Input: part model. Units: mm. Frame: model coordinates. Face numbers are marked on the shaded views. A direction names the side the tool comes from. Give positions to 0.01 mm unless a question says otherwise; leave off trailing zeros. Loops run counter-clockwise (first coordinate to the right, second up) from the corner with the lowest first, then second, coordinate; pieces in that order, holes last. Notation, with made-up numbers: M 41,56.25 L 71,56.25 A13 ccw 71,69.25 Z; hole C 79,-7 d3. An arc over 180 degrees is marked long. Return JSON: item names as keys, results as strings. Group by question number.
Autodesk Inventor part; units mm, degrees
ref_plane "YZ Plane" through (0, 0, 0) normal (1, 0, 0) x (0, 1, 0)
ref_plane "XZ Plane" through (0, 0, 0) normal (0, 1, 0) x (-1, 0, 0)
ref_plane "XY Plane" through (0, 0, 0) normal (0, 0, 1) x (1, 0, 0)
sketch "Sketch1" plane through (0, 0, 0) normal (0, 1, 0) x (-1, 0, 0)
  circle A0 centre (19.9072, 0) radius 5
  line L0 (-15.0928, 12) -> (34.9072, 12)
  line L1 (34.9072, 12) -> (34.9072, -12)
  line L2 (34.9072, -12) -> (-15.0928, -12)
  line L3 (-15.0928, -12) -> (-15.0928, 12)
  point P0 (0, 0)
  dimension "d0" = 10
  dimension "d1" = 12
  dimension "d2" = 24
  dimension "d3" = 35
  dimension "d4" = 50
extrude "Extrusion1" add sketch "Sketch1" along normal blind 10
sketch "Sketch2" plane through (15.0928, 0, 12) normal (1, 0, 0) x (0, 0, -1)
  line L0 (12, 0) -> (12, -23) construction
  line L1 (12, -23) -> (-0.5, -23) construction
  circle A0 centre (-0.5, -23) radius 3
  line L2 (31, 10) -> (-7, 10)
  line L3 (-7, 10) -> (-7, -33)
  line L4 (-7, -33) -> (31, -33)
  line L5 (31, -33) -> (31, 10)
  line L6 (31, 10) -> (-7, -33) construction
  line L7 (-7, 10) -> (31, -33) construction
  circle A1 centre (24.5, -23) radius 3
  point P0 (12, -11.5)
  dimension "d7" = 6
  dimension "d8" = 12.5
extrude "Extrusion2" add sketch "Sketch2" against normal blind 10
chamfer "Chamfer1" distance 15 angle 45 1 edges at (5.0928, 0, 0)
sketch "Sketch3" plane through (-34.9072, 0, -12) normal (-1, 0, 0) x (0, 0, 1)
  circle A0 centre (12, 5) radius 2.95
  line L0 (0, 10) -> (24, 10)
  point P0 (12, 0)
  dimension "d14" = 5.9
  dimension "d15" = 5
extrude "Extrusion3" cut sketch "Sketch3" against normal blind 16
properties part number "Mitutoyo holder"
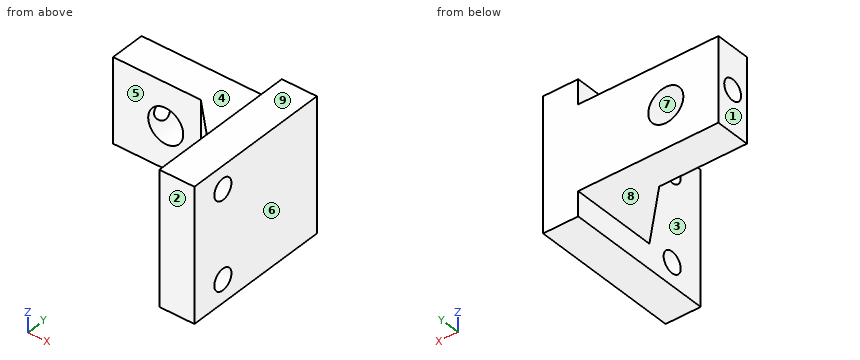
Item 1: Section A-A, the plane y = -23. Return loops of the section in (x, z).
Item 2: Section C-C, the plane z = 8. Return loops of the section in (x, y).
Item 3: Reachability of the marked faces 1, 2, 3, 4 and 5 from +Z, -Z, +X, -X, +Y, -Y: full face, straight path, thin tool, end or side. Return the list, or none.
Item 4: Material intervals for line 1 (Y direction, x = -27.25, z = 0); line 2 (Z direction, x = -31, y = 5); line 3 (Y direction, x = 10.5, z = -12.5), sorted ascending. Write a range as from..to.
Item 5: First-contact query: pin 1 Ø19 at (x, z) = (-18, 4) entering from -Y; pin 2 Ø20 at (x, y) = (-23.5, -6) entering from -Z; pin 3 Ø16 at (x, z) = (-19.91, 0) entering from -Y. Flat tips, straight axial feed; report the tip coordinate or a pass-through.
Item 6: Section B-B, the plane z = 14.5. Return loops of the section in (x, y), then the cut area to 3 significant figures.
Item 7: Section D-D, the plane z = -2. Return loops of the section in (x, y).
Item 8: Pull-direction query (Z, two-part tool) for the marked faces 6, 7, 8 and 9; classes: pulls with the +Z half, pulls with the -Z half, needs draft (parallel to the pull), parting line crosses it, or undercut.
Answer below:
{
 "1": {"outline": "M 5.09,-19 L 15.09,-19 L 15.09,-15.5 L 5.09,-15.5 Z; M 5.09,-9.5 L 15.09,-9.5 L 15.09,9.5 L 5.09,9.5 Z; M 5.09,15.5 L 15.09,15.5 L 15.09,19 L 5.09,19 Z"},
 "2": {"outline": "M -34.91,0 L -9.91,0 L 5.09,-15 L 5.09,-33 L 15.09,-33 L 15.09,10 L -34.91,10 Z"},
 "3": {"face 1": "+Z, -Z, -X, +Y, -Y", "face 2": "+Z, -Z, +X, -X, -Y", "face 3": "-X, -Y", "face 4": "+Z, -X, +Y, -Y", "face 5": "+Z, -Z, -X, -Y"},
 "4": {"line 1": "0..2.05, 7.95..10", "line 2": "-12..-2.95, 2.95..12", "line 3": "-33..-26, -20..10"},
 "5": {"pin 1": "y = -1.41", "pin 2": "z = -12", "pin 3": "y = 0"},
 "6": {"outline": "M 5.09,-33 L 15.09,-33 L 15.09,-25.24 L 5.09,-25.24 Z; M 5.09,-20.76 L 15.09,-20.76 L 15.09,10 L 5.09,10 Z", "area": "385 mm^2"},
 "7": {"outline": "M -34.91,0 L -24.49,0 L -24.49,2.83 L -34.91,2.83 Z; M -34.91,7.17 L -24.49,7.17 L -24.49,10 L -34.91,10 Z; M -15.32,0 L -9.91,0 L 5.09,-15 L 5.09,-33 L 15.09,-33 L 15.09,10 L -15.32,10 Z"},
 "8": {"face 6": "needs draft", "face 7": "undercut", "face 8": "pulls with the -Z half", "face 9": "pulls with the +Z half"}
}
